Build history of the part. All positions in model axes, mm. Coordinates: 2 decimals unless noted, no trailing zeros.
(1) Flat gauge pin, fed straight in: P1, Ø3.5, axis at x = -60.325, z = -9.525, coming from the -Y side (3 decimals). Where does the tip first touch, or does it go through?
(2) Wall check: L1, parallel to X at y = -0.5, z = 10.5; L2, parallel to X at y = -1.75, z = 10.5. Give the ranges that are in metal, low to high.
(3) Two-plate mould, pull along X, no slides. Class faces 1 (the face through (-63.5, 0, 0)), 2 (the face through (58.727, 0.809, 9.455)), 3 (the face through (-61.5, 0.81, 8.44)), 4 (the face through (-1, 0, -15.875)): pulls with the +X half, pulls with the -X half, needs draft (parallel to the pull), parting line crosses it, or undercut.
from build123d import *

# Parameters (mm, degrees)
SKETCH1_W                                       = 127
SKETCH1_H                                       = 31.75
BOSS_EXTRUDE1_DEPTH                             = 3.175
CSK_FOR_M3_FLAT_HEAD_MACHINE_SCREW1_D           = 3.2
CSK_FOR_M3_FLAT_HEAD_MACHINE_SCREW1_DEPTH       = 12.7
CSK_FOR_M3_FLAT_HEAD_MACHINE_SCREW1_CSINK_D     = 6.3
CSK_FOR_M3_FLAT_HEAD_MACHINE_SCREW1_CSINK_ANGLE = 90
CSK_FOR_M3_FLAT_HEAD_MACHINE_SCREW1_TIP         = 0.96137699


with BuildPart() as part:
    # Sketch1 → Boss-Extrude1 (new, symmetric)
    with BuildSketch(Plane(origin=(0, 0, 0), x_dir=(1, 0, 0), z_dir=(0, 1, 0))):
        Rectangle(SKETCH1_W, SKETCH1_H)
    extrude(amount=BOSS_EXTRUDE1_DEPTH, both=True)

    # CSK for M3 Flat Head Machine Screw1
    with Locations(Plane(origin=(0, -3.175, 0), x_dir=(-1, 0, 0), z_dir=(0, -1, 0))):
        with Locations((60.325, -9.525), (60.325, 9.525), (-60.325, -9.525), (-60.325, 9.525)):
            CounterSinkHole(CSK_FOR_M3_FLAT_HEAD_MACHINE_SCREW1_D / 2, CSK_FOR_M3_FLAT_HEAD_MACHINE_SCREW1_CSINK_D / 2, depth=CSK_FOR_M3_FLAT_HEAD_MACHINE_SCREW1_DEPTH, counter_sink_angle=CSK_FOR_M3_FLAT_HEAD_MACHINE_SCREW1_CSINK_ANGLE)
            with Locations((0, 0, -(CSK_FOR_M3_FLAT_HEAD_MACHINE_SCREW1_DEPTH + CSK_FOR_M3_FLAT_HEAD_MACHINE_SCREW1_TIP / 2))):  # 118° drill point
                Cone(0, CSK_FOR_M3_FLAT_HEAD_MACHINE_SCREW1_D / 2, CSK_FOR_M3_FLAT_HEAD_MACHINE_SCREW1_TIP, mode=Mode.SUBTRACT)


solid = part.part
Response values:
1. P1: stops at y = -1.775
2. L1: x = -63.5 to -61.59, -59.06 to 59.06, 61.59 to 63.5
2. L2: x = -63.5 to -61.75, -58.9 to 58.9, 61.75 to 63.5
3. face 1: pulls with the -X half
3. face 2: undercut
3. face 3: undercut
3. face 4: needs draft
